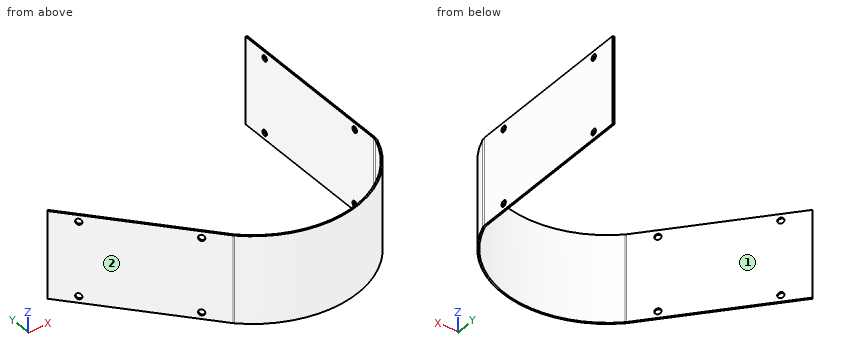
Autodesk Inventor part; units mm, degrees
ref_plane "YZ Plane" through (0, 0, 0) normal (1, 0, 0) x (0, 1, 0)
ref_plane "XZ Plane" through (0, 0, 0) normal (0, 1, 0) x (-1, 0, 0)
ref_plane "XY Plane" through (0, 0, 0) normal (0, 0, 1) x (1, 0, 0)
sketch "Sketch1" plane through (0, 0, 0) normal (0, 0, 1) x (1, 0, 0)
  arc A0 (66.7702, 112.6298) -> (73.6141, 138.1061) centre (52.5264, 130.1136) ccw construction
  line L0 (63.1006, 61.9455) -> (112.0149, 5.088)
  arc A1 (66.7702, 112.6298) -> (63.1006, 61.9455) centre (88.8254, 85.558) ccw construction
  arc A2 (138.8831, 162.8706) -> (162.2319, 146.2144) centre (163.0457, 172.0484) ccw construction
  arc A3 (172.0845, 144.47) -> (162.2319, 146.2144) centre (161.1324, 111.3067) ccw construction
  line L1 (196.0564, 111.0477) -> (195.4211, 25.3647)
  arc A4 (112.0149, 5.088) -> (112.3757, 4.7043) centre (116.5302, 8.9726) ccw
  arc A5 (112.3757, 4.7043) -> (195.1395, 23.7862) centre (147.6111, 40.9044) ccw
  arc A6 (195.1395, 23.7862) -> (195.4211, 25.3647) centre (190.6588, 25.4) ccw
  arc A7 (196.0564, 111.0477) -> (172.0845, 144.47) centre (161.1324, 111.3067) ccw construction
  arc A8 (138.8831, 162.8706) -> (73.6141, 138.1061) centre (105.8063, 151.6542) ccw construction
  line L2 (111.4132, 4.5704) -> (62.5072, 61.4182)
  arc A9 (66.2689, 113.2452) -> (62.5072, 61.4182) centre (88.8254, 85.558) ccw construction
  arc A10 (66.2689, 113.2452) -> (72.8769, 137.8116) centre (52.5264, 130.1136) ccw construction
  arc A11 (139.6302, 163.1392) -> (72.8769, 137.8116) centre (105.8063, 151.6542) ccw construction
  arc A12 (139.6302, 163.1392) -> (162.2569, 147.0077) centre (163.0457, 172.0484) ccw construction
  arc A13 (172.3334, 145.2237) -> (162.2569, 147.0077) centre (161.1324, 111.3067) ccw construction
  arc A14 (196.8501, 111.0418) -> (172.3334, 145.2237) centre (161.1324, 111.3067) ccw construction
  line L3 (196.8501, 111.0418) -> (196.2148, 25.3588)
  arc A15 (195.8863, 23.5172) -> (196.2148, 25.3588) centre (190.6588, 25.4) ccw
  arc A16 (111.8221, 4.1355) -> (195.8863, 23.5172) centre (147.6111, 40.9044) ccw
  arc A17 (111.4132, 4.5704) -> (111.8221, 4.1355) centre (116.5302, 8.9726) ccw
  line L4 (196.0564, 111.0477) -> (196.8501, 111.0418)
  line L5 (63.1006, 61.9455) -> (62.5072, 61.4182)
  point P0 (0, 0)
  point P1 (93.7791, 184.445)
  point P2 (71.0776, 147.9379)
  point P3 (60.2024, 105.5589)
  point P4 (195.6522, 56.526)
  point P5 (134.0244, 172.2363)
  dimension "d0" = 0.7937
extrude "Extrusion1" add sketch "Sketch1" along normal blind 42.164
sketch "Sketch2" plane through (63.1006, 61.9455, 42.164) normal (0.7580738, 0.6521688, 0) x (0, 0, -1)
  line L0 (42.164, 0) -> (42.164, -75.0025)
  line L1 (42.164, 0) -> (0, 0)
  line L2 (0, -75.0025) -> (0, 0)
  line L3 (42.164, -75.0025) -> (0, -75.0025)
  line L4 (3.175, 0) -> (3.175, -75.0025) construction
  line L5 (38.989, 0) -> (38.989, -75.0025) construction
  line L6 (42.164, -62.3025) -> (0, -62.3025) construction
  line L7 (0, -12.7) -> (42.164, -12.7) construction
  point P0 (42.164, -5.807)
  point P1 (3.175, -12.7)
  point P2 (38.989, -12.7)
  point P3 (3.175, -62.3025)
  point P4 (38.989, -62.3025)
  dimension "d4" = 3.175
  dimension "d5" = 3.175
  dimension "d6" = 12.7
  dimension "d7" = 12.7
hole "Hole1" at (71.3831, 52.3179, 38.989) at (71.3831, 52.3179, 3.175) at (103.7323, 14.7156, 38.989) at (103.7323, 14.7156, 3.175) direction (-0.7580738, -0.6521688, 0) diameter 2.9464 depth 25.4 tip angle 118
sketch "Sketch3" plane through (195.4211, 25.3647, 0) normal (-0.9999725, 0.0074143, 0) x (0, 0, 1)
  line L0 (0, 0) -> (0, 85.6854)
  line L1 (0, 0) -> (42.164, 0)
  line L2 (42.164, 85.6854) -> (42.164, 0)
  line L3 (0, 85.6854) -> (42.164, 85.6854)
  line L4 (3.175, 85.6854) -> (3.175, 0) construction
  line L5 (0, 12.7) -> (42.164, 12.7) construction
  line L6 (38.989, 85.6854) -> (38.989, 0) construction
  line L7 (0, 72.9854) -> (42.164, 72.9854) construction
  point P0 (0, -26.8129)
  point P1 (3.175, 72.9854)
  point P2 (38.989, 72.9854)
  point P3 (38.989, 12.7)
  point P4 (3.175, 12.7)
  dimension "d15" = 3.175
  dimension "d16" = 3.175
  dimension "d17" = 12.7
  dimension "d18" = 12.7
hole "Hole2" at (195.9623, 98.3481, 3.175) at (195.9623, 98.3481, 38.989) at (195.5153, 38.0643, 38.989) at (195.5153, 38.0643, 3.175) direction (0.9999725, -0.0074143, 0) diameter 2.9464 depth 25.4 tip angle 118
equation "\"d5\" = d4"
properties part number "Sheild"
Source: CAD feature listing. Evaluate the final solid. Frame: model axes, mm. Face numbers are marked on the shaded views. A direction names the side the tool comes from. Coordinates: 2 decimals unless noted, no trailing zeros. Write each loop counter-clockwise with the first axis right and the second up, starting at its lowest first coordinate (ties: lowest second). Pieces come first, ordered by that corner, then holes. Notation, with made-up numbers: (-3, 23) - (26, 23) arc R23 ccw to (26, 36) - close; hole circle Ø7 at (77, -21). An arc over 180 degrees is marked (long way). Answer as a JSON object with one key per item and string values.
Q1. Section query C-C, the plane y = 31.5. Output: boundary loops of the cut face in (x, z), plus the area to 3 significant figures.
Ans:
{"outline": "(88.25, 0) - (89.29, 0) - (89.29, 42.16) - (88.25, 42.16) - close; (195.47, 0) - (196.26, 0) - (196.26, 42.16) - (195.47, 42.16) - close", "area": "77.6 mm2"}
Q2. Set-up query: the marked faces 1 and 2. Return all of +Z, -Z, +X, -X, +Y, -Y with unobstructed straight access to the full face (end or side cutting, diameter ignored); none if empty.
Ans:
{"face 1": "+Z, -Z, +Y", "face 2": "+Z, -Z, -X, -Y"}
Q3. Section query B-B, the plane z = 14. Output: boundary loops of the cut face in (x, y).
Ans:
{"outline": "(62.51, 61.42) - (111.41, 4.57) arc R6.78 ccw to (111.82, 4.14) arc R51.31 ccw to (195.89, 23.52) arc R5.55 ccw to (196.21, 25.36) - (196.85, 111.04) - (196.06, 111.05) - (195.42, 25.36) arc R4.76 cw to (195.14, 23.79) arc R50.52 cw to (112.38, 4.7) arc R5.97 cw to (112.01, 5.09) - (63.1, 61.95) - close"}
Q4. Material intervals for line 1 (X direction, y = 8, z = 24); line 2 (X direction, y = 26.5, z = 4.5); line 3 (Y direction, x = 147.5, z = 20), sorted ascending. Write a range as [from, to].
Ans:
{"line 1": "x = [108.46, 109.51], [185.94, 186.98]", "line 2": "x = [92.55, 93.59], [195.43, 196.22]", "line 3": "y = [-10.41, -9.61]"}
Q5. Section query A-A, the plane y = 1.5. Output: boundary loops of the cut face in (x, z), plus the area to 3 significant figures.
Ans:
{"outline": "(114.75, 0) - (116, 0) - (116, 42.16) - (114.75, 42.16) - close; (179.22, 0) - (180.48, 0) - (180.48, 42.16) - (179.22, 42.16) - close", "area": "106 mm2"}
Q6. Section query D-D, the plane x = 144. Output: boundary loops of the cut face in (y, z), plus the area to 3 significant figures.
Ans:
{"outline": "(-10.28, 0) - (-9.48, 0) - (-9.48, 42.16) - (-10.28, 42.16) - close", "area": "33.6 mm2"}
Q7. First-contact query: pin 1 Ø4 at (y, z) = (72.5, 16.5) entering from -X; pin 2 Ø12 at (x, z) = (95, 28) entering from -Y; pin 3 Ø10 at (x, z) = (140, 9) entering from -Y. Flat tips, straight axial feed; report the tip coordinate or a pass-through.
Ans:
{"pin 1": "stops at x = 195.76", "pin 2": "stops at y = 16.67", "pin 3": "stops at y = -10.34"}
